Design review of the part built by this model. Coordinates are the model's own, in mm. A direction names the side the tool comes from. Coordinates: 2 decimals unless noted, no trailing zeros. Loops run counter-clockwise (first coordinate to the right, second up) from the corner with the lowest first, then second, coordinate; pieces in that order, holes last. Notation, with made-up numbers: M 51.5,38.25 L 62.5,38.25 A35 ccw 62.5,75.25 Z; hole C 48.5,62.25 d10. An arc over 180 degrees is marked long. Write item = value, one per line. Start each with the question number.
Autodesk Inventor part; units mm, degrees
ref_plane "YZ Plane" through (0, 0, 0) normal (1, 0, 0) x (0, 1, 0)
ref_plane "XZ Plane" through (0, 0, 0) normal (0, 1, 0) x (-1, 0, 0)
ref_plane "XY Plane" through (0, 0, 0) normal (0, 0, 1) x (1, 0, 0)
sketch "Sketch1" plane through (0, 0, 0) normal (0, 0, 1) x (1, 0, 0)
  line L0 (0, 0) -> (-56.9976, 0)
  line L1 (-56.9976, 0) -> (-56.9976, 38.1)
  line L2 (-56.9976, 38.1) -> (0, 38.1)
  line L3 (0, 38.1) -> (0, 0)
  line L4 (0, 38.1) -> (-7.493, 38.1)
  line L5 (-7.493, 38.1) -> (-7.493, 8.1026)
  line L6 (-56.9976, 38.1) -> (-49.5046, 38.1)
  line L7 (-49.5046, 38.1) -> (-49.5046, 8.1026)
  dimension "d1" = 56.9976
  dimension "d2" = 38.1
  dimension "d3" = 7.493
  dimension "d4" = 29.9974
  dimension "d5" = 7.493
extrude "Plate1" add sketch "Sketch1" along normal blind 3.175
sketch "Sketch8" plane through (0, 0, 3.175) normal (0, 0, 1) x (1, 0, 0)
  circle A0 centre (-7.5, 7.9) radius 3.3
  circle A1 centre (-49.5, 7.9) radius 3.3
extrude "Cut1" cut sketch "Sketch8" against normal blind 3.175
sketch "Sketch10" plane through (0, 0, 3.175) normal (1, 0, 0) x (0, 0, -1)
  line L0 (0, 38.1) -> (0, 0)
  line L1 (3.175, 0) -> (0, 0)
  line L2 (3.175, 0) -> (3.175, 38.1)
  line L3 (3.175, 38.1) -> (0, 38.1)
extrude "Extrusion1" add sketch "Sketch10" along normal blind 52.1462
sketch "Sketch13" plane through (0, 38.1, 3.175) normal (0, 1, 0) x (1, 0, 0)
  line L0 (0, 3.175) -> (0, 0)
  line L1 (0, 0) -> (52.1462, 0)
  line L2 (52.1462, 3.175) -> (52.1462, 0)
  line L3 (0, 3.175) -> (52.1462, 3.175)
extrude "Extrusion2" add sketch "Sketch13" along normal blind 76.2
sketch "Sketch14" plane through (0, 0, 0) normal (0, 0, -1) x (-1, 0, 0)
  circle A0 centre (-33.6026, 107.95) radius 3.3782
  circle A1 centre (-33.6026, 92.075) radius 3.3782
  point P0 (0, 0)
extrude "Cut4" cut sketch "Sketch14" against normal blind 3.175
sketch "Sketch15" plane through (0, 0, 3.175) normal (0, 0, 1) x (1, 0, 0)
  line L0 (0, 114.3) -> (52.1462, 114.3)
  line L1 (0, 38.1) -> (0, 114.3)
  line L2 (-56.9976, 38.1) -> (0, 38.1)
  line L3 (52.1462, 114.3) -> (14.0462, 114.3)
  line L4 (14.0462, 114.3) -> (14.0462, 38.1)
  line L5 (14.0462, 38.1) -> (0, 38.1)
  point P0 (0, 0)
  dimension "d31" = 38.1
extrude "Cut5" cut sketch "Sketch15" against normal blind 3.175
equation "\"d19\" = Thickness"
equation "\"d29\" = Thickness"
equation "\"d32\" = Thickness"
equation "\"BendRadius\" = Thickness"
equation "\"BendReliefWidth\" = Thickness"
equation "\"BendReliefDepth\" = 0.5 * Thickness"
equation "\"CornerReliefSize\" = 4 * Thickness"
equation "\"MinimumRemnant\" = 2 * Thickness"
equation "\"TransitionRadius\" = BendRadius"
equation "\"JacobiRadiusSize\" = BendRadius"
equation "\"GapSize\" = Thickness"
equation "\"d8\" = BendRadius"
properties part number "endstop 3" material "Aluminum 6061"
Q1. Add section C-C on y = 7.9. State the section outline as (x, z) points (3 decimals), plus the area to 3 significant figures.
Q2. Mouldability with a two-part tool opening along Y and no side actions: class faces 3 (the face through (-9.93, 10.13, 1.61)), 4 (the face through (-3, 0, 2)), 5 (the face through (-56.998, 19, 2)), 6 (the face through (-22, 38.1, 2)) as released by +Y, released by -Y, zero draft, split by the parting line, or undercut.
Q3. Add section B-B on y = 107.95. State the section outline as (x, z) points (3 decimals).
Q4. Add section A-A on x = -7.5. State the section outline as (y, z) points (3 decimals), plus the area to 3 significant figures.
Q5. To check wall thickness, follow line 1 (Y direction, x = -49.5, z = 1.8); line 2 (Y direction, x = 32.5, z = 2.8); line 3 (Y direction, x = 13, z = 0.65). State the ranges of each line that lie inside material, in increasing order. Write a range as from..to.
Q6. For faces 1 (the face through (30.482, 90.781, 1.565)), 2 (the face through (14.046, 77, 2)), list the 3-axis set-ups (+Z, -Z, +X, -X, +Y, -Y) from which the entire face can be reached by the end or side of a thin tool; tool diameter is ignored.
Q7. Clearance check with flat-ended pins moving along their axes: P1, Ø1.6, axis at y = 57.5, z = 1, coming from the -X side; P2, Ø1.6, axis at x = -7.5, z = 2, coming from the +Y side. State where each tip first meets the part, or that it passes through.
Q8. Add section D-D on z = 1.8. State the section outline as (x, y) points (3 decimals), plus the area to 3 significant figures.
Values follow:
q1.outline = M -56.998,0 L -52.8,0 L -52.8,3.175 L -56.998,3.175 Z; M -46.2,0 L -10.8,0 L -10.8,3.175 L -46.2,3.175 Z; M -4.2,0 L 52.146,0 L 52.146,3.175 L -4.2,3.175 Z
q1.area = 305 mm2
q2.face_3 = undercut
q2.face_4 = released by -Y
q2.face_5 = zero draft
q2.face_6 = released by +Y
q3.outline = M 14.046,0 L 30.224,0 L 30.224,3.175 L 14.046,3.175 Z; M 36.981,0 L 52.146,0 L 52.146,3.175 L 36.981,3.175 Z
q4.outline = M 0,0 L 4.6,0 L 4.6,3.175 L 0,3.175 Z; M 11.2,0 L 38.1,0 L 38.1,3.175 L 11.2,3.175 Z
q4.area = 100 mm2
q5.line_1 = 0..4.6, 11.2..38.1
q5.line_2 = 0..88.88, 95.27..104.76, 111.14..114.3
q5.line_3 = 0..38.1
q6.face_1 = +Z, -Z
q6.face_2 = +Z, -Z, -X, +Y
q7.P1 = 14.05
q7.P2 = 38.1
q8.outline = M -56.998,0 L 52.146,0 L 52.146,114.3 L 14.046,114.3 L 14.046,38.1 L -56.998,38.1 Z; hole C -49.5,7.9 d6.6; hole C -7.5,7.9 d6.6; hole C 33.603,92.075 d6.756; hole C 33.603,107.95 d6.756
q8.area = 6,920 mm2
